Autodesk Inventor part; units mm, degrees
ref_plane "Work Plane2" through (14.3627, 1.55, 6) normal (0, 0, 1) x (1, 0, 0)
ref_plane "YZ Plane" through (0, 0, 0) normal (1, 0, 0) x (0, 1, 0)
ref_plane "XZ Plane" through (0, 0, 0) normal (0, 1, 0) x (-1, 0, 0)
ref_plane "Work Plane1" through (0, -12.9, 0) normal (0, 0, 1) x (1, 0, 0)
sketch "Sketch1" plane through (0, -12.9, 0) normal (0, 0, 1) x (1, 0, 0)
  circle A0 centre (26.8127, 14) radius 1.4 construction
  line L0 (6.8127, 27.5) -> (46.8127, 27.5)
  line L1 (46.8127, 27.5) -> (46.8127, 0.5)
  line L2 (46.8127, 0.5) -> (6.8127, 0.5)
  line L3 (6.8127, 0.5) -> (6.8127, 27.5)
  line L4 (6.8127, 27.5) -> (46.8127, 0.5) construction
  line L5 (46.8127, 27.5) -> (6.8127, 0.5) construction
  circle A1 centre (26.8127, 14) radius 12.7 construction
  circle A2 centre (26.8127, 14) radius 12.85
  line L6 (6.8127, 27.5) -> (46.8127, 27.5)
  line L7 (46.8127, 27.5) -> (46.8127, 28.5)
  line L8 (46.8127, 28.5) -> (6.8127, 28.5)
  line L9 (6.8127, 28.5) -> (6.8127, 27.5)
  point P0 (0, 12.9)
  dimension "d0" = 40
  dimension "d1" = 27
  dimension "d14" = 1
  dimension "d25" = 25.7
ref_plane "Work Plane2" through (14.3627, 1.55, 6) normal (0, 0, 1) x (1, 0, 0)
extrude "Extrusion1" add sketch "Sketch1" along normal up to surface (6 mm away)
ref_plane "Work Plane3" through (11.8127, 24, 6) normal (-1, 0, 0) x (0, 0, 1)
sketch "Sketch2" plane through (11.8127, 24, 6) normal (-1, 0, 0) x (0, 0, 1)
  line L0 (-13.2187, 0) -> (3.0119, 0)
  line L1 (-6, -35.75) -> (-6, -10.05)
  line L2 (-10.9, -34.4) -> (0.6933, -34.4)
  line L3 (-10.9, -31.4) -> (0.6933, -31.4)
  line L4 (-10.9, -14.4) -> (0.6933, -14.4)
  line L5 (-10.9, -11.4) -> (0.6933, -11.4)
  arc A0 (-5.3, -10.45) -> (-5.3, -15.35) centre (-5.3, -12.9) ccw
  arc A1 (-5.4335, -30.45) -> (-5.4335, -35.35) centre (-5.4335, -32.9) ccw
  line L6 (-5.4335, -35.35) -> (-5.4335, -30.45)
  line L7 (-5.3, -15.35) -> (-5.3, -10.45)
  point P0 (-6, -24)
  dimension "d22" = 4.9
  dimension "d23" = 1.5
  dimension "d24" = 1.5
revolve "Revolution1" cut sketch "Sketch2" angle 360 about axis through (11.8127, 8.65, 0.7) along (0, 1, 0) contours A0 L4 L1 | L1 L4 L7 A0 | L4 A0 L5 L1 | L1 L5 L7 L4 | L5 A0 L1 | L1 A0 L7 L5
pattern_linear "Rectangular Pattern1" count 2 spacing 20 along (0, -1, 0) count 2 spacing 30 along (1, 0, 0) of "Revolution1"
sketch "Sketch3" plane through (6.8127, -12.4, 6) normal (0, 0, 1) x (1, 0, 0)
  ellipse E0 centre (20, 24.3) end of major axis (41.0718, 24.3) minor radius 14.9 (7.3193, 12.4) -> (20, 9.4) ccw construction
  ellipse E1 centre (20, 24.3) end of major axis (41.0718, 24.3) minor radius 14.9 (20, 9.4) -> (32.6807, 12.4) ccw construction
  circle A0 centre (20, 13.5) radius 12.85 construction
  line L0 (40, 0) -> (0, 0) construction
  line L1 (40, 28) -> (40, 0) construction
  line L2 (0, 28) -> (40, 28) construction
  line L3 (0, 0) -> (0, 28) construction
  circle A1 centre (20, 13.5) radius 12.85 construction
  line L4 (40, 0) -> (0, 0)
  line L5 (10.0003, 0) -> (29.9997, 0)
  spline S0 degree 5 poles (2.3021, 2.9833) (5.5467, 1.2547) (9.0339, -0.0186) (12.6471, -0.8521) (16.3235, -1.2698) (20, -1.2699) knots 0 0 0 0 0 0 1 1 1 1 1 1
  spline S1 degree 5 poles (20, -1.2699) (23.6765, -1.2698) (27.3529, -0.8521) (30.9661, -0.0186) (34.4533, 1.2547) (37.6979, 2.9833) knots 0 0 0 0 0 0 1 1 1 1 1 1
  point P0 (-6.8127, 12.4)
extrude "Extrusion2" add sketch "Sketch3" against normal up to surface (6 mm away)
ref_plane "Work Plane4" through (26.8127, 23.9, 43.6151) normal (-0.7071068, 0, 0.7071068) x (-0.7071068, 0, -0.7071068)
sketch "Sketch4" plane through (26.8127, 23.9, 43.6151) normal (-0.7071068, 0, 0.7071068) x (-0.7071068, 0, -0.7071068)
  arc A0 (33.8666, 23.9) -> (15.9334, 23.9) centre (24.9, 12) ccw
  ellipse E0 centre (26.5979, 22.8) end of major axis (26.5979, 35.65) minor radius 9.0863 construction
  line L0 (12.4558, 36.3) -> (19.5271, 36.3) construction
  line L1 (12.4558, 8.3) -> (12.4558, 36.3) construction
  line L2 (40.74, 8.3) -> (12.4558, 8.3) construction
  line L3 (40.74, 36.3) -> (40.74, 8.3) construction
  line L4 (33.6687, 36.3) -> (40.74, 36.3)
  arc A1 (33.5545, 36.3) -> (9.1298, 32.4131) centre (24.9, 12) ccw
  line L5 (33.6687, 36.3) -> (40.74, 36.3)
  line L6 (33.5545, 36.3) -> (40.74, 36.3)
  line L7 (40.74, 36.3) -> (40.74, 42.5179)
  line L8 (40.74, 42.5179) -> (9.2813, 42.9694)
  line L9 (9.2813, 42.9694) -> (9.1298, 32.4131)
  point P0 (49.8, 23.9)
extrude "Extrusion3" cut sketch "Sketch4" against normal through all
ref_plane "Work Plane5" through (62.0266, 23.9, 8.4012) normal (0.7071068, 0, 0.7071068) x (-0.7071068, 0, 0.7071068)
sketch "Sketch5" plane through (62.0266, 23.9, 8.4012) normal (0.7071068, 0, 0.7071068) x (-0.7071068, 0, 0.7071068)
  arc A0 (33.8666, 23.9) -> (15.9334, 23.9) centre (24.9, 12) ccw
  arc A1 (40.4723, 32.6668) -> (9.3277, 32.6668) centre (24.9, 12) ccw
  line L0 (16.1313, 36.3) -> (11.8886, 36.3)
  line L1 (16.1313, 36.3) -> (16.2449, 36.3865) construction
  line L2 (16.2449, 36.3865) -> (16.1313, 36.3)
  line L3 (40.4723, 32.6668) -> (40.4723, 41.9024)
  line L4 (40.4723, 41.9024) -> (12.0732, 41.9024)
  line L5 (12.0732, 41.9024) -> (11.8886, 36.3)
  point P0 (37.9189, 23.9)
extrude "Extrusion4" cut sketch "Sketch5" against normal through all
properties part number "20_Cube_Insert_Kinematic_Mirrormount_45_Thorlabsadapter"
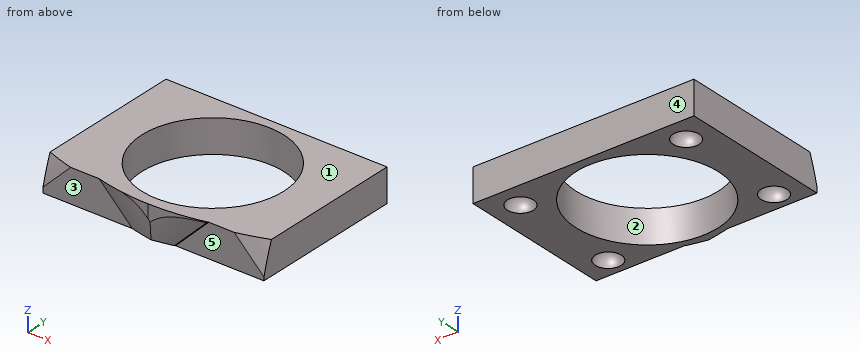
Work out the finished part from the listing and answer in its coordinate system (mm). Face numbers are marked on the shaded views. A direction names the side the tool comes from. Round coordinates to 2 decimals unless told otherwise and drop trailing zeros. Write each loop counter-clockwise with the first axis right and the second up, starting at its lowest first coordinate (ties: lowest second). Pieces come first, ordered by that corner, then holes.
1) A cutting plane is placed at A-A (y = 1.1). Give the vertices of the cut face in (x, z), plus the area to 3 significant figures.
2) Straight lines are drawn through the part: line 1 (X direction, y = 0.75, z = 2.5); line 2 (Y direction, x = 27, z = 3.5); line 3 (Y direction, x = 9.5, z = 2.75). For each, find the intervals that lie inside material, in ascending order.
3) A cutting plane is placed at C-C (z = 2). Give the number of separate pieces and of enclosed holes in the cut face, plus the area to 3 significant figures.
4) A cutting plane is placed at D-D (y = -2). Give the vertices of the cut face in (x, z).
5) The mould has two halves that part along Y. Classify the marked faces 1, 2 and 3: pulls with the +Y half, pulls with the -Y half, needs draft (parallel to the pull), parting line crosses it, or undercut.
6) Given pin 1 Ø1.8 at (x, z) = (41.5, 1.5) entering from -Y, flat-ended and moving along its own axis, determine where the tip first touches the part or whether it passes through.
7) A cutting plane is placed at B-B (y = -9.75). Give the vertices of the cut face in (x, z), plus the area to 3 significant figures.
8) A tool of negligible diameter and unlimited length cuts with its end or side. For the marked faces 4 and 5, from which of +Z, -Z, +X, -X, +Y, -Y can it reach the whole face along a straight path? Write none if from no direction.
Completed:
1. outline: (6.81, 0) - (13.96, 0) - (13.96, 6) - (6.81, 6) - close; (39.66, 0) - (46.81, 0) - (46.81, 6) - (39.66, 6) - close
1. area: 85.8 mm2
2. line 1: x = 6.81 to 13.97, 39.66 to 46.81
2. line 2: y = -13.67 to -11.75, 13.95 to 15.6
2. line 3: y = -12.4 to 15.6
3. separate pieces: 1
3. enclosed holes: 5
3. area: 554 mm2
4. outline: (6.81, 0) - (14.34, 0) - (14.34, 6) - (6.81, 6) - close; (39.28, 0) - (46.81, 0) - (46.81, 6) - (39.28, 6) - close
5. face 1: needs draft
5. face 2: undercut
5. face 3: pulls with the -Y half
6. pin 1: stops at y = -12.4
7. outline: (6.81, 0) - (9.62, 0) arc R2.3 cw (long way) to (14, 0) - (19.93, 0) - (19.93, 6) - (6.81, 6) - close; (33.7, 0) - (39.62, 0) arc R2.3 cw (long way) to (44, 0) - (46.81, 0) - (46.81, 6) - (33.7, 6) - close
7. area: 134 mm2
8. face 4: +Z, -Z, +X, -X, +Y
8. face 5: -Z, +X, -Y
